Input: part model. Units: mm. Frame: model coordinates. A direction names the side the tool comes from. Coordinates: 2 decimals unless noted, no trailing zeros. Loops run counter-clockwise (first coordinate to the right, second up) from the corner with the lowest first, then second, coordinate; pieces in that order, holes last.
```python
from build123d import *

# Parameters (mm, degrees)
F1_DEPTH  = 6.35
F3_DEPTH  = 24.13
F4_W      = 101.6
F4_H      = 6.35
F5_DEPTH  = 6.35
F7_DEPTH  = 12.7
F8_W      = 9.525
F8_H      = 2.54
F9_DEPTH  = 114.282591
F10_W     = 9.525
F10_H     = 2.54
F11_DEPTH = 12.7
F13_DEPTH = 12.7
F19_DEPTH = 44.196
F21_DEPTH = 2.54
F23_DEPTH = 2.54
F24_R     = 3.81
F25_DEPTH = 6.35
F26_W     = 2.9521
F26_H     = 3.065642
F27_DEPTH = 20.5232


with BuildPart() as f1:
    # F0 (on Front) → F1 (new body)
    with BuildSketch(Plane.XZ):
        with BuildLine():
            Line((0, 25.4), (0, 0))
            Line((0, 0), (25.4, 0))
            Line((25.4, 0), (25.4, 25.4))
            ThreePointArc((25.4, 25.4), (12.7, 38.1), (0, 25.4))
        make_face()
    extrude(amount=F1_DEPTH)

    # F2 (on face) → F3 (join)
    with BuildSketch(Plane(origin=(0, 0, 0), x_dir=(1, 0, 0), z_dir=(0, 0, -1))):
        Polygon((-4.953, 3.175), (0, 0), (0, 6.35), align=None)
        Polygon((30.353, 3.175), (25.4, 6.35), (25.4, 0), align=None)
    extrude(amount=-F3_DEPTH)

    # F4 (on face) → F5 (join)
    with BuildSketch(Plane(origin=(0, 0, 0), x_dir=(1, 0, 0), z_dir=(0, 0, -1))):
        with Locations((12.7, 3.175)):
            Rectangle(F4_W, F4_H)
    extrude(amount=F5_DEPTH)

    # F6 (on face) → F7 (join)
    with BuildSketch(Plane.XZ.offset(6.35)):
        Polygon((25.4, 0), (0, 0), (-38.1, 0), (-38.1, -6.35), (63.5, -6.35), (63.5, 0), align=None)
    extrude(amount=F7_DEPTH)

    # F8 (on face) → F9 (cut)
    with BuildSketch(Plane.YZ.offset(63.5)):
        with Locations((-11.1125, -1.27)):
            Rectangle(F8_W, F8_H)
    extrude(amount=-F9_DEPTH, mode=Mode.SUBTRACT)

    # F18 (on face) + F17 (on face) → F19 (join)
    with BuildSketch(Plane.XY):
        Polygon((63.5, 0), (58.42, -3.175), (63.5, -6.35), align=None)
    with BuildSketch(Plane.XY):
        Polygon((-33.02, -3.175), (-38.1, 0), (-38.1, -6.35), align=None)
    extrude(amount=F19_DEPTH)

    # F20 (on face) → F21 (join)
    with BuildSketch(Plane(origin=(-38.1, 0, 0), x_dir=(0, -1, 0), z_dir=(-1, 0, 0))):
        Polygon((6.35, -2.54), (6.35, 0), (6.35, 44.196), (0, 44.196), (0, 0), (0, -6.35), (6.35, -6.35), align=None)
    extrude(amount=F21_DEPTH)

    # F22 (on face) → F23 (join)
    with BuildSketch(Plane.YZ.offset(63.5)):
        Polygon((-6.35, 0), (-6.35, -2.54), (-6.35, -6.35), (0, -6.35), (0, 0), (0, 44.196), (-6.35, 44.196), align=None)
    extrude(amount=F23_DEPTH)

    # F24 (on face) → F25 (join)
    with BuildSketch(Plane(origin=(0, 0, 0), x_dir=(-1, 0, 0), z_dir=(0, 1, 0))):
        with Locations((-12.7, 25.4)):
            Circle(F24_R)
    extrude(amount=F25_DEPTH)

    # F26 (on Right) → F27 (cut)
    with BuildSketch(Plane.YZ):
        with Locations((2.497112, 21.865308)):
            Rectangle(F26_W, F26_H)
    extrude(amount=F27_DEPTH, mode=Mode.SUBTRACT)


with BuildPart() as f11:
    # F10 (on face) → F11 (new body)
    with BuildSketch(Plane.YZ.offset(63.5)):
        with Locations((-11.1125, -1.27)):
            Rectangle(F10_W, F10_H)
    extrude(amount=F11_DEPTH)


with BuildPart() as f13:
    # F12 (on face) → F13 (new body)
    with BuildSketch(Plane.YZ.offset(63.5)):
        Polygon((-6.35, -6.35), (-6.35, -2.54), (-15.875, -2.54), (-15.875, 0), (-19.05, 0), (-19.05, -6.35), align=None)
    extrude(amount=F13_DEPTH)


solid = f1.part
```
Item 1: Line query: L1, parallel to Y at x = -24.5, z = -2 (3 decimals); L2, parallel to Z at x = -2.5, y = -13.5; L3, parallel to Z at x = -10.5, y = -1.75. Output: solid intervals per line, ascending.
Result:
L1: y = -19.05 to -15.875, -6.35 to 0
L2: z = -6.35 to -2.54
L3: z = -6.35 to 0
Item 2: Section query A-A (z = 3.5). Output: boundary loops of the cut face in (x, y) (3 decimals).
Result:
outline: (-40.64, -6.35) - (-38.1, -6.35) - (-33.02, -3.175) - (-38.1, 0) - (-40.64, 0) - close; (-4.953, -3.175) - (0, -6.35) - (25.4, -6.35) - (30.353, -3.175) - (25.4, 0) - (0, 0) - close; (58.42, -3.175) - (63.5, -6.35) - (66.04, -6.35) - (66.04, 0) - (63.5, 0) - close
Item 3: Section query B-B (x = 12.7). Output: boundary loops of the cut face in (y, z) (3 decimals).
Result:
outline: (-19.05, -6.35) - (0, -6.35) - (0, 21.59) - (1.021, 21.59) - (1.021, 23.398) - (3.973, 23.398) - (3.973, 21.59) - (6.35, 21.59) - (6.35, 29.21) - (0, 29.21) - (0, 38.1) - (-6.35, 38.1) - (-6.35, -2.54) - (-15.875, -2.54) - (-15.875, 0) - (-19.05, 0) - close
Item 4: Reachability of faces 1 (the face through (-2.442, -4.785, 11.896)), 2 (the face through (-2.51, -1.61, 11.9)), 3 (the face through (-2, -3, 24.13)), 4 (the face through (63.5, -14, -4)), 5 (the face through (13, -15.875, -1)) from +Z, -Z, +X, -X, +Y, -Y: full face, straight path, thin tool, end or side. Return the list, or none.
Result:
face 1: +Z, -Y
face 2: +Z, +Y
face 3: +Z, +Y, -Y
face 4: +Z, -Z, +X, -Y
face 5: +Z, +X, -X
Item 5: Section query D-D (x = 52.5). Output: boundary loops of the cut face in (y, z) (3 decimals), then the cut area to 3 significant figures.
Result:
outline: (-19.05, -6.35) - (0, -6.35) - (0, 0) - (-6.35, 0) - (-6.35, -2.54) - (-15.875, -2.54) - (-15.875, 0) - (-19.05, 0) - close
area: 96.8 mm2
Item 6: Mould query, pull axis Y, two halves, no side actions, for faces 6 (the face through (13, -11, -2.54)), 7 (the face through (-35.524, -1.61, 21.789)), 8 (the face through (12, -6.35, 15)), 9 (the face through (13, -17, 0)). Classes: +Y half, -Y half, draft (parallel to the pull), parting line (faces both ways), or undercut.
Result:
face 6: undercut
face 7: +Y half
face 8: undercut
face 9: draft
Item 7: Contact query for flat-ended pins moving along their axis: P1, Ø4, axis at x = 20, z = 3.5, coming from the +Y side; P2, Ø5, axis at y = -10, z = -2.5, coming from the +X side; P3, Ø0.5, axis at x = 12, z = 22.5, coming from the -Y side; P4, Ø2, axis at x = -29, z = 2.5, coming from the +Y side. Output: stop coordinate, or through.
Result:
P1: stops at y = 0
P2: stops at x = 63.5
P3: stops at y = -6.35
P4: passes through
Item 8: Section query C-C (y = 2.75). Output: boundary loops of the cut face in (x, z), then the cut area to 3 significant figures.
Result:
outline: (9.46, 23.4) - (15.94, 23.4) arc R3.81 ccw (long way) to start
area: 37.3 mm2
